```python
from build123d import *

# Parameters (mm, degrees)
BOSS_EXTRUDE1_DEPTH     = 10
SKETCH2_R               = 2.6
CUT_EXTRUDE1_DEPTH      = 142.774468788
SKETCH3_W               = 60
SKETCH3_H               = 9
SKETCH3_W_2             = 9
SKETCH3_H_2             = 60
BOSS_EXTRUDE3_DEPTH     = 1.46
CUT_EXTRUDE2_DEPTH      = 142.774468788
CUT_EXTRUDE2_DEPTH_BACK = 142.774468788
SKETCH2_2_R             = 2.6
CHAMFER1_SIZE           = 1.46
CUT_EXTRUDE3_START      = 10
SKETCH4_R               = 4.5
CUT_EXTRUDE3_DEPTH      = 5
SKETCH5_W               = 100
SKETCH5_H               = 50
BOSS_EXTRUDE4_DEPTH     = 5
BOSS_EXTRUDE5_DEPTH     = 10
BOSS_EXTRUDE6_START     = 100
BOSS_EXTRUDE6_DEPTH     = 10
CUT_EXTRUDE4_DEPTH      = 154.622914957
CUT_EXTRUDE4_DEPTH_BACK = 154.622914957
SKETCH10_R              = 1.75
CUT_EXTRUDE5_START      = 100
SKETCH11_R              = 3.5
CUT_EXTRUDE5_DEPTH      = 95
SKETCH12_W              = 10
SKETCH12_H              = 5
SKETCH12_W_2            = 5
SKETCH12_H_2            = 10
CUT_EXTRUDE6_DEPTH      = 5
CHAMFER2_SIZE           = 5


# Some blends are built 0.0001 mm under size
with BuildPart() as part:
    # Sketch1 → Boss-Extrude1 (new body)
    with BuildSketch(Plane.XY):
        Polygon((0, 0), (100, 0), (100, 40), (20, 100), (0, 100), align=None)
    extrude(amount=BOSS_EXTRUDE1_DEPTH)

    # Sketch2 → Cut-Extrude1 (cut, through all)
    with BuildSketch(Plane.XY):
        with Locations((10, 85)):
            Circle(SKETCH2_R)
        with Locations((10, 60)):
            Circle(SKETCH2_R)
        with Locations((85, 30)):
            Circle(SKETCH2_R)
        with Locations((85, 10)):
            Circle(SKETCH2_R)
        with Locations((60, 10)):
            Circle(SKETCH2_R)
        with Locations((60, 30)):
            Circle(SKETCH2_R)
    extrude(amount=CUT_EXTRUDE1_DEPTH, mode=Mode.SUBTRACT)

    # Sketch3 → Boss-Extrude3 (add)
    with BuildSketch(Plane.XY):
        with Locations((70, 30)):
            Rectangle(SKETCH3_W, SKETCH3_H)
        with Locations((70, 10)):
            Rectangle(SKETCH3_W, SKETCH3_H)
        with Locations((10, 70)):
            Rectangle(SKETCH3_W_2, SKETCH3_H_2)
    extrude(amount=-BOSS_EXTRUDE3_DEPTH)

    # Sketch2<2> → Cut-Extrude2 (cut, two sides: drawn at the far end of the back side and taken through both)
    with BuildSketch(Plane.XY.offset(-CUT_EXTRUDE2_DEPTH_BACK)):
        with Locations((10, 85)):
            Circle(SKETCH2_2_R)
        with Locations((10, 60)):
            Circle(SKETCH2_2_R)
        with Locations((85, 30)):
            Circle(SKETCH2_2_R)
        with Locations((85, 10)):
            Circle(SKETCH2_2_R)
        with Locations((60, 10)):
            Circle(SKETCH2_2_R)
        with Locations((60, 30)):
            Circle(SKETCH2_2_R)
    extrude(amount=CUT_EXTRUDE2_DEPTH + CUT_EXTRUDE2_DEPTH_BACK, mode=Mode.SUBTRACT)

    # Chamfer1
    chamfer1_edges = [part.edges().sort_by_distance(p)[0] for p in [
        (14.5, 70, -1.46),
        (5.5, 70, -1.46),
        (70, 5.5, -1.46),
        (70, 14.5, -1.46),
        (70, 25.5, -1.46),
        (70, 34.5, -1.46),
    ]]
    chamfer(chamfer1_edges, length=CHAMFER1_SIZE - 0.0001)  # a hair under: the kernel refuses the full size

    # Sketch4 → Cut-Extrude3 (cut)
    with BuildSketch(Plane.XY.offset(CUT_EXTRUDE3_START)):
        with Locations((10, 85)):
            Circle(SKETCH4_R)
        with Locations((10, 60)):
            Circle(SKETCH4_R)
        with Locations((60, 30)):
            Circle(SKETCH4_R)
        with Locations((85, 30)):
            Circle(SKETCH4_R)
        with Locations((85, 10)):
            Circle(SKETCH4_R)
        with Locations((60, 10)):
            Circle(SKETCH4_R)
    extrude(amount=-CUT_EXTRUDE3_DEPTH, mode=Mode.SUBTRACT)

    # Sketch5 → Boss-Extrude4 (add)
    with BuildSketch(Plane(origin=(0, 0, 0), x_dir=(1, 0, 0), z_dir=(0, 1, 0))):
        with Locations((50, -35)):
            Rectangle(SKETCH5_W, SKETCH5_H)
    extrude(amount=BOSS_EXTRUDE4_DEPTH)

    # Sketch8 → Boss-Extrude5 (add)
    with BuildSketch(Plane(origin=(0, 0, 0), x_dir=(0, 0, -1), z_dir=(1, 0, 0))):
        Polygon((-10, 5), (-60, 5), (-10, 40), align=None)
    extrude(amount=BOSS_EXTRUDE5_DEPTH)

    # Sketch8<2> → Boss-Extrude6 (add)
    with BuildSketch(Plane(origin=(0, 0, 0), x_dir=(0, 0, -1), z_dir=(1, 0, 0)).offset(BOSS_EXTRUDE6_START)):
        Polygon((-10, 5), (-60, 5), (-10, 40), align=None)
    extrude(amount=-BOSS_EXTRUDE6_DEPTH)

    # Sketch10 → Cut-Extrude4 (cut, two sides: drawn at the far end of the back side and taken through both)
    with BuildSketch(Plane(origin=(0, 0, 0), x_dir=(1, 0, 0), z_dir=(0, 1, 0)).offset(-CUT_EXTRUDE4_DEPTH_BACK)):
        with Locations(Location((5, -50, 0), (0, 0, 270))):
            Circle(SKETCH10_R)
        with Locations(Location((95, -50, 0), (0, 0, 270))):
            Circle(SKETCH10_R)
        with Locations(Location((95, -15, 0), (0, 0, 270))):
            Circle(SKETCH10_R)
        with Locations(Location((5, -15, 0), (0, 0, 270))):
            Circle(SKETCH10_R)
    extrude(amount=CUT_EXTRUDE4_DEPTH + CUT_EXTRUDE4_DEPTH_BACK, mode=Mode.SUBTRACT)

    # Sketch11 → Cut-Extrude5 (cut)
    with BuildSketch(Plane(origin=(0, 0, 0), x_dir=(1, 0, 0), z_dir=(0, 1, 0)).offset(CUT_EXTRUDE5_START)):
        with Locations(Location((5, -15, 0), (0, 0, 270))):
            Circle(SKETCH11_R)
        with Locations(Location((5, -50, 0), (0, 0, 270))):
            Circle(SKETCH11_R)
        with Locations(Location((95, -50, 0), (0, 0, 270))):
            Circle(SKETCH11_R)
        with Locations(Location((95, -15, 0), (0, 0, 270))):
            Circle(SKETCH11_R)
    extrude(amount=-CUT_EXTRUDE5_DEPTH, mode=Mode.SUBTRACT)

    # Sketch12 → Cut-Extrude6 (cut)
    with BuildSketch(Plane(origin=(0, 0, 0), x_dir=(1, 0, 0), z_dir=(0, 1, 0))):
        with Locations((50, -57.5)):
            Rectangle(SKETCH12_W, SKETCH12_H)
        with Locations((97.5, -30)):
            Rectangle(SKETCH12_W_2, SKETCH12_H_2)
        with Locations((2.5, -30)):
            Rectangle(SKETCH12_W_2, SKETCH12_H_2)
    extrude(amount=CUT_EXTRUDE6_DEPTH, mode=Mode.SUBTRACT)

    # Chamfer2
    # the kernel refuses this chamfer: 5 mm, written as the material it takes off along each edge
    with BuildSketch(Plane(origin=(3.333333333, 96.666666667, 6.666666667), x_dir=(-0.7071067811865474, 0, -0.7071067811865476), z_dir=(-0.5773502691896258, 0.5773502691896257, 0.5773502691896257))) as chamfer2_piece_1:
        Polygon((-3.535533906, 2.041241452), (3.535533906, 2.041241452), (0, -4.082482905), align=None)
    extrude(amount=6.350852961, mode=Mode.SUBTRACT)
    with BuildSketch(Plane(origin=(110.286731952, 32.284951036, 10), x_dir=(0.016497525966350957, 0.021996701288467948, -0.9996219169112968), z_dir=(-0.8000000000000002, 0.6, 0))) as chamfer2_piece_2_section:
        Polygon((CHAMFER2_SIZE * 0.999621916911, CHAMFER2_SIZE * 0.0274958766106), (-CHAMFER2_SIZE * 0.0274958766106, CHAMFER2_SIZE * 0.999621916911), (0, 0), align=None)
    chamfer2_piece_2 = extrude(amount=125.71682988, mode=Mode.PRIVATE)
    chamfer2_piece_2 = split(chamfer2_piece_2, bisect_by=Plane(origin=(56.438385269, 50.830938552, -5.472769359), z_dir=(0, 0.8192319205190406, 0.5734623443633283)), keep=Keep.TOP, mode=Mode.PRIVATE)
    add(chamfer2_piece_2, mode=Mode.SUBTRACT)
    with BuildSketch(Plane(origin=(100, -12.85841494, 60), x_dir=(0.0274958766105877, 0, -0.9996219169112968), z_dir=(0, 1, 0))) as chamfer2_piece_3:
        Polygon((CHAMFER2_SIZE * 0.999621916911, CHAMFER2_SIZE * 0.0274958766106), (-CHAMFER2_SIZE * 0.0274958766106, CHAMFER2_SIZE * 0.999621916911), (0, 0), align=None)
    extrude(amount=30.71682988, mode=Mode.SUBTRACT)
    with BuildSketch(Plane(origin=(0, -12.85841494, 60), x_dir=(-0.027495876610586372, 0, -0.9996219169112968), z_dir=(0, 1, 0))) as chamfer2_piece_4:
        Polygon((CHAMFER2_SIZE * 0.999621916911, -CHAMFER2_SIZE * 0.0274958766106), (-CHAMFER2_SIZE * 0.0274958766106, -CHAMFER2_SIZE * 0.999621916911), (0, 0), align=None)
    extrude(amount=30.71682988, mode=Mode.SUBTRACT)
    with BuildSketch(Plane(origin=(32.85841494, 100, 10), x_dir=(0, 0.0274958766105877, -0.9996219169112968), z_dir=(-1, 0, 0))) as chamfer2_piece_5:
        Polygon((CHAMFER2_SIZE * 0.999621916911, CHAMFER2_SIZE * 0.0274958766106), (-CHAMFER2_SIZE * 0.0274958766106, CHAMFER2_SIZE * 0.999621916911), (0, 0), align=None)
    extrude(amount=45.71682988, mode=Mode.SUBTRACT)
    with BuildSketch(Plane(origin=(0, 112.85841494, 10), x_dir=(-0.02749587661058638, 0, -0.9996219169112968), z_dir=(0, -1, 0))) as chamfer2_piece_6_section:
        Polygon((CHAMFER2_SIZE * 0.999621916911, CHAMFER2_SIZE * 0.0274958766106), (-CHAMFER2_SIZE * 0.0274958766106, CHAMFER2_SIZE * 0.999621916911), (0, 0), align=None)
    chamfer2_piece_6 = extrude(amount=85.71682988, mode=Mode.PRIVATE)
    chamfer2_piece_6 = split(chamfer2_piece_6, bisect_by=Plane(origin=(1.674929178, 50.830938552, -5.472769359), z_dir=(0, 0.8192319205190406, 0.5734623443633283)), keep=Keep.TOP, mode=Mode.PRIVATE)
    add(chamfer2_piece_6, mode=Mode.SUBTRACT)
    with BuildSketch(Plane(origin=(0, 100, -12.85841494), x_dir=(-0.027495876610586313, -0.9996219169112968, 0), z_dir=(0, 0, 1))) as chamfer2_piece_7:
        Polygon((CHAMFER2_SIZE * 0.999621916911, CHAMFER2_SIZE * 0.0274958766106), (-CHAMFER2_SIZE * 0.0274958766106, CHAMFER2_SIZE * 0.999621916911), (0, 0), align=None)
    extrude(amount=35.71682988, mode=Mode.SUBTRACT)


solid = part.part
```
Build history of the part. All positions in model axes, mm. A direction names the side the tool comes from. Coordinates: 2 decimals unless noted, no trailing zeros. Order: outer loops, then holes, each group sorted by start corner. A loop starts at its lowest first (then second) coordinate and runs counter-clockwise, first axis right, second up.
Item 1: Drop flat-ended pins along their axis: pin 1 Ø4.5 at (x, y) = (85, 29) entering from +Z; pin 2 Ø1.6 at (y, z) = (11, -1) entering from -X; pin 3 Ø7 at (x, y) = (85, 11.5) entering from +Z. Give the stop position or say it passes through.
Filled in:
pin 1: stops at z = 5
pin 2: stops at x = 40
pin 3: stops at z = 10
Item 2: Saw through at A-A on z = 50. List the corners of the cut face in (x, y).
Filled in:
outline: (0, 0) - (3.25, 0) - (3.25, 5) - (1.5, 5) - (1.5, 12) - (0, 12) - close; (6.75, 0) - (93.25, 0) - (93.25, 5) - (91.5, 5) - (91.5, 12) - (90, 12) - (90, 5) - (10, 5) - (10, 12) - (8.5, 12) - (8.5, 5) - (6.75, 5) - close; (96.75, 0) - (100, 0) - (100, 12) - (98.5, 12) - (98.5, 5) - (96.75, 5) - close
Item 3: Drill centre lines: L1, parallel to X at y = 30, z = 2.5; L2, parallel to Z at x = 5, y = 10.25; L3, parallel to X at y = 30.5, z = 9. Where is each one in solid material? Low to high.
Filled in:
L1: x = 0 to 57.4, 62.6 to 82.4, 87.6 to 100
L2: z = 0 to 11.5, 18.5 to 46.5
L3: x = 0 to 55.53, 64.47 to 80.53, 89.47 to 100
Item 4: Tool access for faces 5 (the flat face through (12, 83, 5)), 6 (the flat face through (2, 2, 35)), 7 (the flat face through (4, 5, 13)): list every direction of +Z, -Z, +X, -X, +Y, -Y with a clear straight run to the whole face (end or side of a thin tool).
Filled in:
face 5: +Z
face 6: -X, -Y
face 7: +Y
Item 5: Mould opens along X. For faces 1 (the flat face through (70, 10, -1.46)), 2 (the cylindrical face through (9.662, 87.578, 1.725)), 3 (the flat face through (87, 8, 5)), 4 (the flat face through (5, 2, 30)) say: released by +X, released by -X, zero draft, split by the parting line, or undercut.
Filled in:
face 1: zero draft
face 2: undercut
face 3: undercut
face 4: released by -X
Item 6: Saw through at C-C on y = 30. List the corners of the cut face in (x, z).
Filled in:
outline: (0, 0) - (40, 0) - (40, -1.46) - (57.4, -1.46) - (57.4, 5) - (55.5, 5) - (55.5, 10) - (10, 10) - (10, 24.29) - (0, 24.29) - close; (62.6, -1.46) - (82.4, -1.46) - (82.4, 5) - (80.5, 5) - (80.5, 10) - (64.5, 10) - (64.5, 5) - (62.6, 5) - close; (87.6, -1.46) - (100, -1.46) - (100, 24.29) - (90, 24.29) - (90, 10) - (89.5, 10) - (89.5, 5) - (87.6, 5) - close; hole circle Ø7 at (5, 15); hole circle Ø7 at (95, 15)
